The listing builds one solid part. Answer for the finished solid, in the listing's coordinates (mm). A direction names the side the tool comes from. Give positions to 0.01 mm unless a question says otherwise; leave off trailing zeros. Loops run counter-clockwise (first coordinate to the right, second up) from the corner with the lowest first, then second, coordinate; pieces in that order, holes last. Notation, with made-up numbers: (57, 82.25) - (100, 82.25) arc R16 cw to (100, 96.25) - close; hole circle Ø6 at (67, -27). An arc over 180 degrees is marked (long way). Answer in a Markdown table with one row per item. Add a question column.
```python
from build123d import *

# Parameters (mm, degrees)
PAD_DEPTH       = 19.5
SKETCH001_W     = 13.6
SKETCH001_H     = 19.5
POCKET_DEPTH    = 10
POCKET001_DEPTH = 20
POCKET002_DEPTH = 1.7
POCKET003_DEPTH = 1.7
SKETCH005_R     = 1
PAD001_DEPTH    = 1.5
FILLET_R        = 0.3
SKETCH006_R     = 1
PAD002_DEPTH    = 1.5
FILLET001_R     = 0.3
SKETCH007_W     = 1.7
SKETCH007_H     = 6
POCKET004_DEPTH = 20
SKETCH008_W     = 1.7
SKETCH008_H     = 6
POCKET005_DEPTH = 20
SKETCH009_W     = 1.5
SKETCH009_H     = 6
POCKET006_DEPTH = 1.7
FILLET002_R     = 0.3
FILLET003_R     = 0.3
SKETCH010_W     = 1.5
SKETCH010_H     = 6
POCKET007_DEPTH = 1.7
FILLET004_R     = 0.3
FILLET005_R     = 0.3
FILLET006_R     = 0.3
FILLET007_R     = 0.3
FILLET008_R     = 0.7


with BuildPart() as part:
    # Sketch → Pad (new body)
    with BuildSketch(Plane.XY):
        Polygon((-3, 0), (-3, -2.5), (-4.5, -2.5), (-4.5, -4), (4.5, -4), (4.5, -2.5), (3, -2.5), (3, 0), (10, 0), (10, 12), (-10, 12), (-10, 0), align=None)
    extrude(amount=PAD_DEPTH)

    # Sketch001 (on Face10 of Pad) → Pocket (cut)
    with BuildSketch(Plane(origin=(0, 12, 0), x_dir=(-1, 0, 0), z_dir=(0, 1, 0))):
        with Locations((0, 9.75)):
            Rectangle(SKETCH001_W, SKETCH001_H)
    extrude(amount=-POCKET_DEPTH, mode=Mode.SUBTRACT)

    # Sketch002 (on Face6 of Pocket) → Pocket001 (cut)
    with BuildSketch(Plane(origin=(-10, 0, 0), x_dir=(0, -1, 0), z_dir=(-1, 0, 0))):
        with BuildLine():
            ThreePointArc((-2, 14.500024), (-7.000024, 19.5), (-12, 14.499976))
            Line((-12, 14.499976), (-12, 20.5))
            Line((-12, 20.5), (0, 20.5))
            Line((0, 20.5), (0, 14.500024))
            Line((0, 14.500024), (-2, 14.500024))
        make_face()
    extrude(amount=-POCKET001_DEPTH, mode=Mode.SUBTRACT)

    # Sketch003 (on Face8 of Pocket001) → Pocket002 (cut)
    with BuildSketch(Plane(origin=(-10, 0, 0), x_dir=(0, -1, 0), z_dir=(-1, 0, 0))):
        with BuildLine():
            ThreePointArc((-6.999976, 9), (-3.110929, 18.389104), (-12.5, 14.499976))
            Line((-12.5, 14.499976), (-12.5, 9))
            Line((-12.5, 9), (-6.999976, 9))
        make_face()
    extrude(amount=-POCKET002_DEPTH, mode=Mode.SUBTRACT)

    # Sketch004 (on Face14 of Pocket002) → Pocket003 (cut)
    with BuildSketch(Plane.YZ.offset(10)):
        with BuildLine():
            ThreePointArc((12.5, 14.499976), (3.110929, 18.389104), (6.999976, 9))
            Line((12.5, 9), (6.999976, 9))
            Line((12.5, 14.499976), (12.5, 9))
        make_face()
    extrude(amount=-POCKET003_DEPTH, mode=Mode.SUBTRACT)

    # Sketch005 (on Face25 of Pocket003) → Pad001 (join)
    with BuildSketch(Plane.YZ.offset(8.3)):
        with Locations((7, 14.5)):
            Circle(SKETCH005_R)
    extrude(amount=PAD001_DEPTH)

    # Fillet
    fillet_edges = [part.edges().sort_by_distance(p)[0] for p in [
        (9.8, 6, 14.5),
    ]]
    fillet(fillet_edges, radius=FILLET_R)

    # Sketch006 (on Face13 of Fillet) → Pad002 (join)
    with BuildSketch(Plane(origin=(-8.3, 0, 0), x_dir=(0, -1, 0), z_dir=(-1, 0, 0))):
        with Locations((-7, 14.5)):
            Circle(SKETCH006_R)
    extrude(amount=PAD002_DEPTH)

    # Fillet001
    fillet001_edges = [part.edges().sort_by_distance(p)[0] for p in [
        (-9.8, 8, 14.5),
    ]]
    fillet(fillet001_edges, radius=FILLET001_R)

    # Sketch007 (on Face18 of Fillet001) → Pocket004 (cut)
    with BuildSketch(Plane.YZ.offset(10)):
        with Locations((11.15, 4.5)):
            Rectangle(SKETCH007_W, SKETCH007_H)
    extrude(amount=-POCKET004_DEPTH, mode=Mode.SUBTRACT)

    # Sketch008 (on Face18 of Pocket004) → Pocket005 (cut)
    with BuildSketch(Plane.YZ.offset(10)):
        with Locations((7.95, 4.5)):
            Rectangle(SKETCH008_W, SKETCH008_H)
    extrude(amount=-POCKET005_DEPTH, mode=Mode.SUBTRACT)

    # Sketch009 (on Face18 of Pocket005) → Pocket006 (cut)
    with BuildSketch(Plane.YZ.offset(10)):
        with Locations((9.55, 4.5)):
            Rectangle(SKETCH009_W, SKETCH009_H)
    extrude(amount=-POCKET006_DEPTH, mode=Mode.SUBTRACT)

    # Fillet002
    fillet002_edges = [part.edges().sort_by_distance(p)[0] for p in [
        (8.3, 10.3, 4.5),
    ]]
    fillet(fillet002_edges, radius=FILLET002_R)

    # Fillet003
    fillet003_edges = [part.edges().sort_by_distance(p)[0] for p in [
        (8.3, 8.8, 4.5),
    ]]
    fillet(fillet003_edges, radius=FILLET003_R)

    # Sketch010 (on Face26 of Fillet003) → Pocket007 (cut)
    with BuildSketch(Plane(origin=(-10, 0, 0), x_dir=(0, -1, 0), z_dir=(-1, 0, 0))):
        with Locations((-9.55, 4.5)):
            Rectangle(SKETCH010_W, SKETCH010_H)
    extrude(amount=-POCKET007_DEPTH, mode=Mode.SUBTRACT)

    # Fillet004
    fillet004_edges = [part.edges().sort_by_distance(p)[0] for p in [
        (-8.3, 10.3, 4.5),
    ]]
    fillet(fillet004_edges, radius=FILLET004_R)

    # Fillet005
    fillet005_edges = [part.edges().sort_by_distance(p)[0] for p in [
        (-8.3, 8.8, 4.5),
    ]]
    fillet(fillet005_edges, radius=FILLET005_R)

    # Fillet006
    fillet006_edges = [part.edges().sort_by_distance(p)[0] for p in [
        (-9.15, 1.5, 14.500024),
    ]]
    fillet(fillet006_edges, radius=FILLET006_R)

    # Fillet007
    fillet007_edges = [part.edges().sort_by_distance(p)[0] for p in [
        (9.15, 1.5, 14.500024),
    ]]
    fillet(fillet007_edges, radius=FILLET007_R)

    # Fillet008
    fillet008_edges = [part.edges().sort_by_distance(p)[0] for p in [
        (0, 2, 14.500024),
    ]]
    fillet(fillet008_edges, radius=FILLET008_R)


solid = part.part
```
(1) A tool of negligible diameter and unlimited length cuts with its end or side. For faces 5 (the face through (-7, 10.3, 4)), 6 (the face through (7, 8.8, 4)), 7 (the face through (-8.3, 7, 13)), from which of +Z, -Z, +X, -X, +Y, -Y can it reach the whole face along a straight path? Write none if from no direction.
(2) A cutting plane is placed at C-C on x = 4. Determine the outline of the cut face in (y, z).
(3) Given pin 1 Ø3 at (x, z) = (-6.5, 4) entering from +Y; pin 2 Ø0.6 at (x, z) = (7.5, 3.5) entering from -Y; pin 3 Ø1 at (y, z) = (9.5, 5.5) entering from +X, each flat-ended and moving along its own axis, determine where each tip first touches the part or whether it passes through.
(4) A cutting plane is placed at A-A on z = 6.75. Determine the outline of the cut face in (x, y), plus the area to 3 significant figures.
(5) Find the intervals of material crossed by line 1 along X through (y, z) = (4, 11.5); line 2 along Y through (x, z) = (3.25, 10); line 3 along X through (y, z) = (5, 6.75), in increasing order. Write a range as [from, to].
(6) A cutting plane is placed at D-D on x = -0.5. Determine the outline of the cut face in (y, z).
(7) The mould has two halves that part along Y. Classify faces 1 (the face through (0, 0, 17)), 2 (the face through (4, -2.5, 10)), 3 (the face through (7.5, 6.9, 19.5)), 4 (the face through (-9.8, 7, 15)): pulls with the +Y half, pulls with the -Y half, needs draft (parallel to the pull), parting line crosses it, or undercut.
(8) A cutting plane is placed at B-B on y = 8.5. Determine the outline of the cut face in (x, z).
Evaluation:
| question | item | result |
|---|---|---|
| 1 | face 5 | +X, -X, +Y |
| 1 | face 6 | +X, -X |
| 1 | face 7 | -X |
| 2 | outline | (-4, 0) - (-2.5, 0) - (-2.5, 19.5) - (-4, 19.5) - close; (0, 0) - (2, 0) - (2, 13.8) arc R0.7 ccw to (1.3, 14.5) - (0, 14.5) - close |
| 3 | pin 1 | stops at y = 10.3 |
| 3 | pin 2 | stops at y = 0 |
| 3 | pin 3 | stops at x = 8.3 |
| 4 | outline | (-10, 0) - (-3, 0) - (-3, -2.5) - (-4.5, -2.5) - (-4.5, -4) - (4.5, -4) - (4.5, -2.5) - (3, -2.5) - (3, 0) - (10, 0) - (10, 7.1) - (6.8, 7.1) - (6.8, 2) - (-6.8, 2) - (-6.8, 7.1) - (-10, 7.1) - close; (-8.3, 9.1) arc R0.3 ccw to (-8, 8.8) - (-6.8, 8.8) - (-6.8, 10.3) - (-8, 10.3) arc R0.3 ccw to (-8.3, 10) - close; (6.8, 8.8) - (8, 8.8) arc R0.3 ccw to (8.3, 9.1) - (8.3, 10) arc R0.3 ccw to (8, 10.3) - (6.8, 10.3) - close |
| 4 | area | 106 mm² |
| 5 | line 1 | x = [-8.3, -6.8], [6.8, 8.3] |
| 5 | line 2 | y = [-4, -2.5], [0, 2] |
| 5 | line 3 | x = [-10, -6.8], [6.8, 10] |
| 6 | outline | (-4, 0) - (2, 0) - (2, 13.8) arc R0.7 ccw to (1.3, 14.5) - (0, 14.5) - (0, 19.5) - (-4, 19.5) - close |
| 7 | face 1 | pulls with the +Y half |
| 7 | face 2 | undercut |
| 7 | face 3 | parting line crosses it |
| 7 | face 4 | needs draft |
| 8 | outline | (-10, 0) - (-6.8, 0) - (-6.8, 1.5) - (-10, 1.5) - close; (-10, 7.5) - (-6.8, 7.5) - (-6.8, 19.27) - (-8.3, 19.27) - (-8.3, 9) - (-10, 9) - close; (6.8, 0) - (10, 0) - (10, 1.5) - (6.8, 1.5) - close; (6.8, 7.5) - (10, 7.5) - (10, 9) - (8.3, 9) - (8.3, 19.27) - (6.8, 19.27) - close |
